CAD build for the part. Positions are in the model's coordinates, mm. A direction names the side the tool comes from. Give positions to 0.01 mm unless a question says otherwise; leave off trailing zeros. Order: outer loops, then holes, each group sorted by start corner. A loop starts at its lowest first (then second) coordinate and runs counter-clockwise, first axis right, second up. Notation, with made-up numbers: (-11, 3.25) -> (-5, 3.25) arc R22 ccw to (-5, 36.25) -> close; hole circle Ø5 at (35, -19.5). An arc over 180 degrees is marked (long way). Answer as CSV lines item,"result".
Autodesk Inventor part; units mm, degrees
ref_plane "YZ Plane" through (0, 0, 0) normal (1, 0, 0) x (0, 1, 0)
ref_plane "XZ Plane" through (0, 0, 0) normal (0, 1, 0) x (-1, 0, 0)
ref_plane "XY Plane" through (0, 0, 0) normal (0, 0, 1) x (1, 0, 0)
sketch "スケッチ2" plane through (0, 0, 0) normal (0, 1, 0) x (-1, 0, 0)
  line L0 (-35, 0) -> (-18, 0)
  line L1 (-18, -40.5) -> (-18, -65)
  line L2 (-18, -65) -> (0, -65)
  line L3 (0, -65) -> (0, -35)
  line L4 (-18, 0) -> (-68, 0)
  line L5 (-68, 0) -> (-68, -30.5)
  line L6 (-68, -30.5) -> (-28, -30.5)
  line L7 (-18, -30.5) -> (-18, 0)
  arc A0 (0, -35) -> (-35, 0) centre (-35, -35) ccw
  arc A1 (-18, -40.5) -> (-28, -30.5) centre (-28, -40.5) ccw
  point P0 (0, 0)
  point P1 (-38, -10)
  point P2 (-35, 0)
  dimension "d0" = 18
  dimension "d1" = 65
  dimension "d2" = 50
  dimension "d3" = 30.5
  dimension "d18" = 35
  dimension "d19" = 10
extrude "押し出し1" add sketch "スケッチ2" along normal blind 40 contours A0 L3 L2 L1 A1 L6 L5 L4
sketch "スケッチ3" plane through (0, 40, 0) normal (0, 1, 0) x (1, 0, 0)
  line L0 (0, 65) -> (0, 0)
  line L1 (18, 65) -> (0, 65)
  line L2 (14, 48) -> (0, 48) construction
  line L3 (18, 40.5) -> (18, 65) construction
  line L4 (18, 48) -> (0, 48) construction
  line L5 (9, 65) -> (9, 37.3061) construction
  point P0 (4, 48)
  point P1 (0, 32.5)
  point P2 (9, 38)
  point P3 (9, 58)
  point P4 (9, 48)
  dimension "d6" = 4
  dimension "d8" = 17
  dimension "d9" = 17
  dimension "d36" = 10
  dimension "d37" = 10
  dimension "d38" = 4
hole "穴1" at (4, 40, -48) at (14, 40, -48) at (9, 40, -38) at (9, 40, -58) direction (0, -1, 0) diameter 3.3 end through all
fillet "フィレット1" radius 0.5 14 edges at (48, 40, -30.5) (68, 40, -15.25) (0, 40, -50) (18, 40, -52.75) (9, 40, -65) (18, 20, -65) (18, 0, -52.75) (48, 0, -30.5) (68, 20, -30.5) (68, 20, 0) (68, 0, -15.25) (0, 0, -50) (9, 0, -65) (0, 20, -65)
sketch "スケッチ5" plane through (0, 40, 0) normal (0, 1, 0) x (1, 0, 0)
  line L0 (17.5, 64.5) -> (0.5, 64.5)
  line L1 (67.5, 30.5) -> (28, 30.5)
  line L2 (17.5, 64.5) -> (27.5, 64.5)
  line L3 (27.5, 64.5) -> (27.5, 30.5)
  line L4 (27.5, 30.5) -> (17.5, 30.5)
  line L5 (17.5, 30.5) -> (17.5, 64.5)
  line L6 (20.2, 33.7051) -> (20.2, 61.147) construction
  circle A0 centre (14, 48) radius 1.65 construction
  point P0 (0, 0)
  point P1 (20.2, 37.5)
  point P2 (20.2, 58.5)
  dimension "d20" = 6.2
  dimension "d21" = 10
  dimension "d22" = 10.5
  dimension "d23" = 10.5
extrude "押し出し2" [suppressed]
sketch "スケッチ6" plane through (0, 40, 0) normal (0, 1, 0) x (1, 0, 0)
  line L0 (20.2, 39.1303) -> (20.2, 62.5) construction
  line L1 (27.5, 62.5) -> (17.5, 62.5) construction
  circle A0 centre (14, 48) radius 1.65 construction
  point P0 (0, 0)
  point P1 (20.2, 37.5)
  point P2 (20.2, 58.5)
  dimension "d26" = 6.2
  dimension "d27" = 10.5
  dimension "d28" = 10.5
hole "穴2" [suppressed]
properties part number "elbow_stopper" material "ABS プラスチック"
1) Band-saw the part on A-A, the plane y = 27. Write the cut outline in (x, z), then the cut area to 3 significant figures.
Data:
outline,"(0, -64.5) arc R0.5 ccw to (0.5, -65) -> (17.5, -65) arc R0.5 ccw to (18, -64.5) -> (18, -40.5) arc R10 cw to (28, -30.5) -> (67.5, -30.5) arc R0.5 ccw to (68, -30) -> (68, -0.5) arc R0.5 ccw to (67.5, 0) -> (35, 0) arc R35 ccw to (0, -35) -> close; hole circle Ø3.3 at (4, -48); hole circle Ø3.3 at (9, -58); hole circle Ø3.3 at (9, -38); hole circle Ø3.3 at (14, -48)"
area,"2,420 mm2"
2) Band-saw the part on B-B, the plane z = -48. Write the cut outline in (x, y), then the cut area to 3 significant figures.
Data:
outline,"(0, 0.5) arc R0.5 ccw to (0.5, 0) -> (2.35, 0) -> (2.35, 40) -> (0.5, 40) arc R0.5 ccw to (0, 39.5) -> close; (5.65, 0) -> (12.35, 0) -> (12.35, 40) -> (5.65, 40) -> close; (15.65, 0) -> (17.5, 0) arc R0.5 ccw to (18, 0.5) -> (18, 39.5) arc R0.5 ccw to (17.5, 40) -> (15.65, 40) -> close"
area,"456 mm2"
3) Which spindle directions (+Z, -Z, +X, -X, +Y, -Y) get a long thin tool onto all of the face, cutting with end or side? Do faces 5 (the flat face through (68, 20, -15)), 6 (the flat face through (18, 20, -52)). Say none if no direction does.
Data:
face 5,"+Z, -Z, +X, +Y, -Y"
face 6,"-Z, +X, +Y, -Y"
4) Wall check: line 1 along X through (y, z) = (16, -47.5); line 2 along X through (y, z) = (4.5, -41.5); line 3 along X through (y, z) = (36.5, -38.5). Give the ranges that are in metal, low to high. Write a range as [from, to].
Data:
line 1,"x = [0, 2.43], [5.57, 12.43], [15.57, 18]"
line 2,"x = [0, 18]"
line 3,"x = [0, 7.43], [10.57, 18.2]"
5) Band-saw the part on D-D, the plane z = -58. Write the cut outline in (x, y), then the cut area to 3 significant figures.
Data:
outline,"(0, 0.5) arc R0.5 ccw to (0.5, 0) -> (7.35, 0) -> (7.35, 40) -> (0.5, 40) arc R0.5 ccw to (0, 39.5) -> close; (10.65, 0) -> (17.5, 0) arc R0.5 ccw to (18, 0.5) -> (18, 39.5) arc R0.5 ccw to (17.5, 40) -> (10.65, 40) -> close"
area,"588 mm2"
6) Band-saw the part on C-C, the plane x = 54. Write the cut outline in (y, z).
Data:
outline,"(0, -30) arc R0.5 ccw to (0.5, -30.5) -> (39.5, -30.5) arc R0.5 ccw to (40, -30) -> (40, -0.5) arc R0.5 ccw to (39.5, 0) -> (0.5, 0) arc R0.5 ccw to (0, -0.5) -> close"
7) Pin check, flat tips, straight feed: P1, Ø12, axis at y = 34.5, z = -48.5, coming from the +X side; P2, Ø10, axis at x = 26, y = 25, coming from the -Z side; P3, Ø1, axis at y = 32, z = -10, coming from the -X side (3 decimals); P4, Ø3, axis at x = 14, z = -48, coming from the -Y side. Stop position of each tip, or through.
Data:
P1,"stops at x = 18"
P2,"stops at z = -33.36"
P3,"stops at x = 10.005"
P4,"passes through"
8) Pull direction X, two halves, no side cores. Call faces 1 (the flat face through (0, 20, -50)), 2 (the cylindrical face through (21.01, 19.73, -33.35)), 3 (the cylindrical face through (8.93, 19.72, -59.65)), 4 (the flat face through (9, 20, -65)): pulls with the +X half, pulls with the -X half, needs draft (parallel to the pull), parting line crosses it, or undercut.
Data:
face 1,"pulls with the -X half"
face 2,"pulls with the +X half"
face 3,"undercut"
face 4,"needs draft"
